```python
from build123d import *

# Parameters (mm, degrees)
F0_W      = 160.5
F0_H      = 82
F1_DEPTH  = 135
F2_W      = 12.7
F2_H      = 19.05
F2_W_2    = 29.6125
F2_W_3    = 55.0125
F3_DEPTH  = 160.501
F4_W      = 116.05
F4_H      = 19.05
F4_W_2    = 19.05
F4_W_3    = 160.5
F4_H_2    = 38.925
F5_DEPTH  = 12.7
F6_W      = 25.4
F6_H      = 19.05
F6_W_2    = 116.05
F7_DEPTH  = 74.34175
F8_W      = 19.05
F8_H      = 19.05
F9_DEPTH  = 114.58845
F10_SIZE  = 5.08
F11_W     = 28.7067964673
F11_H     = 142.8163200617
F12_DEPTH = 17.65534


with BuildPart() as f1:
    # F0 (on Top) → F1 (new body)
    with BuildSketch(Plane.XY):
        with Locations((80.25, 41)):
            Rectangle(F0_W, F0_H)
    extrude(amount=F1_DEPTH)

    # F2 (on face) → F3 (cut, through all)
    with BuildSketch(Plane.YZ.offset(160.5)):
        with Locations((6.35, 125.475)):
            Rectangle(F2_W, F2_H)
        with Locations((40.20625, 125.475)):
            Rectangle(F2_W_2, F2_H)
        with Locations((74.0625, 125.475)):
            Rectangle(F2_W, F2_H)
        with Locations((74.0625, 9.525)):
            Rectangle(F2_W, F2_H)
        with Locations((27.50625, 9.525)):
            Rectangle(F2_W_3, F2_H)
    extrude(amount=-F3_DEPTH, mode=Mode.SUBTRACT)

    # F4 (on face) → F5 (cut)
    with BuildSketch(Plane(origin=(0, 82, 0), x_dir=(-1, 0, 0), z_dir=(0, 1, 0))):
        with Locations((-102.475, 125.475)):
            Rectangle(F4_W, F4_H)
        with Locations((-9.525, 125.475)):
            Rectangle(F4_W_2, F4_H)
        with Locations((-80.25, 86.9625)):
            Rectangle(F4_W_3, F4_H_2)
        with Locations((-80.25, 48.0375)):
            Rectangle(F4_W_3, F4_H_2)
        with BuildLine():
            Line((-28.575, 135), (-34.925, 135))
            Line((-34.925, 135), (-34.925, 125.475))
            ThreePointArc((-34.925, 125.475), (-31.75, 122.3), (-28.575, 125.475))
            Line((-28.575, 125.475), (-28.575, 135))
        make_face()
        with BuildLine():
            ThreePointArc((-28.575, 9.525), (-31.75, 12.7), (-34.925, 9.525))
            Line((-34.925, 9.525), (-34.925, 0))
            Line((-34.925, 0), (-28.575, 0))
            Line((-28.575, 0), (-28.575, 9.525))
        make_face()
        with Locations((-102.475, 9.525)):
            Rectangle(F4_W, F4_H)
        with Locations((-9.525, 9.525)):
            Rectangle(F4_W_2, F4_H)
    extrude(amount=-F5_DEPTH, mode=Mode.SUBTRACT)

    # F6 (on face) → F7 (cut)
    with BuildSketch(Plane.XZ):
        with Locations((12.7, 125.475)):
            Rectangle(F6_W, F6_H)
        with Locations((102.475, 125.475)):
            Rectangle(F6_W_2, F6_H)
        with Locations((12.7, 9.525)):
            Rectangle(F6_W, F6_H)
        with Locations((102.475, 9.525)):
            Rectangle(F6_W_2, F6_H)
    extrude(amount=-F7_DEPTH, mode=Mode.SUBTRACT)

    # F8 (on face) → F9 (cut)
    with BuildSketch(Plane.YZ.offset(160.5)):
        with Locations((9.525, 106.425)):
            Rectangle(F8_W, F8_H)
        with Locations((72.475, 106.425)):
            Rectangle(F8_W, F8_H)
        with Locations((72.475, 28.575)):
            Rectangle(F8_W, F8_H)
        with Locations((9.525, 28.575)):
            Rectangle(F8_W, F8_H)
    extrude(amount=-F9_DEPTH, mode=Mode.SUBTRACT)

    # F10
    f10_edges = [f1.edges().sort_by_distance(p)[0] for p in [
        (103.205775, 19.05, 96.9),
        (103.205775, 0, 96.9),
        (103.205775, 19.05, 115.95),
        (160.5, 41, 115.95),
        (160.5, 62.95, 28.575),
        (160.5, 66.125, 38.1),
        (160.5, 69.3, 67.5),
        (160.5, 66.125, 96.9),
        (160.5, 62.95, 106.425),
        (160.5, 19.05, 106.425),
        (160.5, 9.525, 96.9),
        (160.5, 0, 67.5),
        (160.5, 9.525, 38.1),
        (160.5, 19.05, 28.575),
        (160.5, 41, 19.05),
        (103.205775, 19.05, 38.1),
        (103.205775, 0, 38.1),
        (103.205775, 19.05, 19.05),
    ]]
    chamfer(f10_edges, length=F10_SIZE)

    # F11 (on face) → F12 (cut)
    with BuildSketch(Plane(origin=(0, 0, 0), x_dir=(0, -1, 0), z_dir=(-1, 0, 0))):
        with Locations((-82.9201973975, 60.9774813056)):
            Rectangle(F11_W, F11_H)
    extrude(amount=-F12_DEPTH, mode=Mode.SUBTRACT)


solid = f1.part
```
The model under review builds one solid part; all positions refer to its coordinate system, in mm. A direction names the side the tool comes from. Give positions to 0.01 mm unless a question says otherwise; leave off trailing zeros. Write each loop counter-clockwise with the first axis right and the second up, starting at its lowest first coordinate (ties: lowest second). Pieces come first, ordered by that corner, then holes. Notation, with made-up numbers: (7.25, 29) - (65.25, 29) arc R23 cw to (65.25, 44) - close; hole circle Ø9 at (11, 20.5). An arc over 180 degrees is marked (long way). Answer in a Markdown table with one row per item. Add a question column.
1. We need section B-B on y = 75. Write out the cut boundary in (x, z) (3 decimals), then the cut area to 3 significant figures.
2. Tool access review of faces 1 (the flat face through (35, 12.7, 125)), 2 (the flat face through (157.92, 60.45, 30.95)), 3 (the flat face through (157.92, 21.55, 106.36)), 4 (the flat face through (44.45, 61, 9)), 5 (the flat face through (25.4, 61, 9)): name each direction out of +Z, -Z, +X, -X, +Y, -Y from which nothing blocks a thin tool from reaching the whole face with its end or side.
3. We need section C-C on y = 16. Write out the cut boundary in (x, z), then the cut area to 3 significant figures.
4. Insertion check: P1, Ø4, axis at x = 100, z = 19.5, coming from the -Y side; P2, Ø4, axis at x = 141.5, y = 51, coming from the -Z side; P3, Ø1, axis at x = 43.5, z = 105, coming from the -Y side; P4, Ø5, axis at x = 25, z = 32.5, coming from the +Y side. Each pin has a flat end and moves straight along its axis. Give the tip position at first contact, or say it passes through.
5. Draft analysis for pull direction Y (two halves, no side actions). For faces 6 (the flat face through (88, 69.3, 68)), 7 (the flat face through (32, 76, 28.575)), 8 (the flat face through (35, 80.412, 123)), 9 (the flat face through (35, 55.012, 9)), state which applies: +Y half, -Y half, draft (parallel to the pull), parting line (faces both ways), or undercut.
6. Wall thickness on line 1 along Z through (x, y) = (18, 77.5) (3 decimals); line 2 along Y through (x, z) = (65, 65): over which ranges is each line inside the solid? List them lowest first. Write a range as [from, to].
7. We need section D-D on z = 95. Write out the cut boundary in (x, y).
Ans:
| question | item | result |
|---|---|---|
| 1 | outline | (17.655, 19.05) - (45.912, 19.05) - (45.912, 28.575) - (17.655, 28.575) - close; (17.655, 106.425) - (45.912, 106.425) - (45.912, 115.95) - (17.655, 115.95) - close |
| 1 | area | 538 mm^2 |
| 2 | face 1 | +Z, +X, -X, -Y |
| 2 | face 2 | -Z, +X, +Y |
| 2 | face 3 | +Z, +X, -Y |
| 2 | face 4 | -Z, +X, +Y, -Y |
| 2 | face 5 | -Z, -X, -Y |
| 3 | outline | (0, 19.05) - (45.91, 19.05) - (45.91, 36.07) - (155.42, 36.07) - (160.5, 41.15) - (160.5, 93.85) - (155.42, 98.93) - (45.91, 98.93) - (45.91, 115.95) - (44.45, 115.95) - (44.45, 135) - (25.4, 135) - (25.4, 115.95) - (0, 115.95) - close |
| 3 | area | 12,000 mm^2 |
| 4 | P1 | stops at y = 21.68 |
| 4 | P2 | stops at z = 19.05 |
| 4 | P3 | stops at y = 0 |
| 4 | P4 | stops at y = 69.3 |
| 5 | face 6 | +Y half |
| 5 | face 7 | draft |
| 5 | face 8 | undercut |
| 5 | face 9 | -Y half |
| 6 | line 1 | z = [19.05, 28.575], [106.425, 115.95] |
| 6 | line 2 | y = [0, 69.3] |
| 7 | outline | (0, 0) - (45.91, 0) - (45.91, 3.18) - (155.42, 3.18) - (157.32, 5.08) - (157.32, 13.97) - (160.5, 17.15) - (160.5, 57.87) - (157.32, 61.05) - (157.32, 67.4) - (155.42, 69.3) - (17.66, 69.3) - (17.66, 68.57) - (0, 68.57) - close |
